from build123d import *

# Parameters (mm, degrees)
F1_DEPTH = 13.97
F2_W     = 12.7
F2_H     = 1.257444
F3_DEPTH = 15.24
F4_W     = 1.27
F4_H     = 1.27
F5_DEPTH = 12.7
F6_W     = 1.27
F6_H     = 1.27
F7_DEPTH = 12.7


with BuildPart() as f1:
    # F0 (on Front) → F1 (new body)
    with BuildSketch(Plane.XZ):
        Polygon((-6.35, 0), (0, 0), (6.35, 0), (6.35, 1.27), (0, 1.27), (-6.35, 1.27), align=None)
    extrude(amount=F1_DEPTH)

    # F2 (on face) → F3 (join)
    with BuildSketch(Plane.XY.offset(1.27)):
        with Locations((0, -0.628722)):
            Rectangle(F2_W, F2_H)
    extrude(amount=F3_DEPTH)

    # F4 (on face) → F5 (join)
    with BuildSketch(Plane(origin=(0, 0, 0), x_dir=(1, 0, 0), z_dir=(0, 0, -1))):
        with Locations((-5.715, 13.335)):
            Rectangle(F4_W, F4_H)
        with Locations((-5.715, 0.635)):
            Rectangle(F4_W, F4_H)
        with Locations((5.715, 0.635)):
            Rectangle(F4_W, F4_H)
        with Locations((5.715, 13.335)):
            Rectangle(F4_W, F4_H)
    extrude(amount=F5_DEPTH)

    # F6 (on face) → F7 (join)
    with BuildSketch(Plane(origin=(0, -12.7, 0), x_dir=(-1, 0, 0), z_dir=(0, 1, 0))):
        with Locations((-5.715, -12.065)):
            Rectangle(F6_W, F6_H)
    extrude(amount=F7_DEPTH)

    # F8: F1 across plane


with BuildPart() as f1_1:
    add(f1.part)
    add(f1.part.mirror(Plane.YZ))


solid = f1_1.part
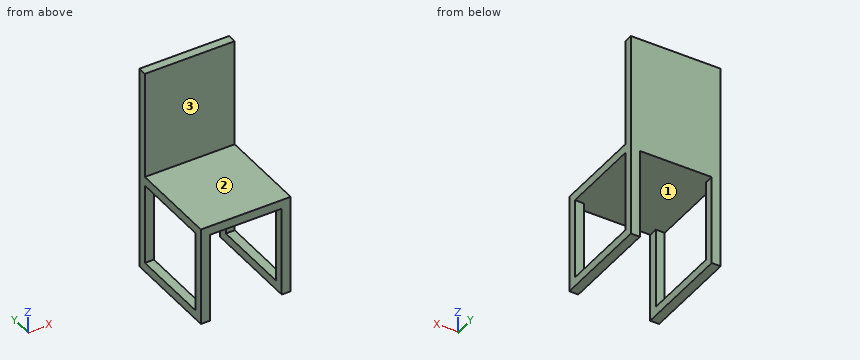
Input: part model. Units: mm. Frame: model coordinates. Face numbers are marked on the shaded views. Coordinates: 2 decimals unless noted, no trailing zeros. Loops run counter-clockwise (first coordinate to the right, second up) from the corner with the lowest first, then second, coordinate; pieces in that order, holes last.
Q1. Cut plane C-C (x = -1.75). Output: boundary loops of the cut face in (y, z), then the cut area to 3 significant figures.
Q2. Cut plane B-B (z = -5). Output: boundary loops of the cut face in (x, y).
Q3. Cut plane D-D (y = -0.75). Output: boundary loops of the cut face in (x, z).
Q4. Draft query along Y for the marked faces 1, 2 and 3. Return one class per face: +Y half, -Y half, draft (parallel to the pull), parting line (faces both ways), or undercut.
Q5. Cut plane A-A (y = -9.25). Output: boundary loops of the cut face in (x, z).
Q6. Material intervals for line 1 (Z direction, x = -5.75, y = -2.25); line 2 (Z direction, x = -2.75, y = -10); line 3 (Y direction, x = -2.75, z = 3.5), sorted ascending.
Q7. Contact query for flat-ended pins moving along their axis: pin 1 (1 mm diameter, centred on x = 6, y = -10, fed in from +Z); pin 2 (2 mm diameter, centred on x = 1, y = -9, fed in from -Z); pin 3 (6.5 mm diameter, centred on x = 2.5, z = 8, fed in from -Y). Output: stop coordinate, or through.
Working result:
1. outline: (-13.97, 0) - (0, 0) - (0, 16.51) - (-1.26, 16.51) - (-1.26, 1.27) - (-13.97, 1.27) - close
1. area: 36.9 mm2
2. outline: (-6.35, -13.97) - (-5.08, -13.97) - (-5.08, -12.7) - (-6.35, -12.7) - close; (-6.35, -1.27) - (-5.08, -1.27) - (-5.08, 0) - (-6.35, 0) - close; (5.08, -13.97) - (6.35, -13.97) - (6.35, -12.7) - (5.08, -12.7) - close; (5.08, -1.27) - (6.35, -1.27) - (6.35, 0) - (5.08, 0) - close
3. outline: (-6.35, -12.7) - (-5.08, -12.7) - (-5.08, 0) - (5.08, 0) - (5.08, -12.7) - (6.35, -12.7) - (6.35, 16.51) - (-6.35, 16.51) - close
4. face 1: undercut
4. face 2: draft
4. face 3: -Y half
5. outline: (-6.35, -12.7) - (-5.08, -12.7) - (-5.08, -11.43) - (-6.35, -11.43) - close; (-6.35, 0) - (6.35, 0) - (6.35, 1.27) - (-6.35, 1.27) - close; (5.08, -12.7) - (6.35, -12.7) - (6.35, -11.43) - (5.08, -11.43) - close
6. line 1: z = -12.7 to -11.43, 0 to 1.27
6. line 2: z = 0 to 1.27
6. line 3: y = -1.26 to 0
7. pin 1: stops at z = 1.27
7. pin 2: stops at z = 0
7. pin 3: stops at y = -1.26
